```python
from build123d import *

# Parameters (mm, degrees)
F1_DEPTH = 18
F2_R     = 15
F4_D     = 8
F4_DEPTH = 15
F4_TIP   = 2.4034424761
F6_DEPTH = 18


# Not quite as in the source:
# - a feature names something its author has since deleted; it is built from what else it names


with BuildPart() as f1:
    # F0 (on Top) → F1 (new body)
    with BuildSketch(Plane.XY):
        Polygon((1700, 0), (0, 0), (0, -750), (1690, -750), (1700, -750), align=None)
    extrude(amount=F1_DEPTH)

    # F2
    f2_edges = [f1.edges().sort_by_distance(p)[0] for p in [
        (0, -750, 9),
        (0, 0, 9),
        (1700, 0, 9),
    ]]
    fillet(f2_edges, radius=F2_R)

    # F4
    with Locations(Plane(origin=(0, 0, 0), x_dir=(1, 0, 0), z_dir=(0, 0, -1))):
        with Locations((136.6116523517, 286.6116523517), (100, 250), (100, 375), (136.6116523517, 463.3883476483), (100, 500), (313.3883476483, 463.3883476483), (350, 375), (313.3883476483, 286.6116523517), (1200, 150), (1450, 150), (1589.5405845398, 110.4594154602), (1600, 250), (1450, 375), (1200, 375), (1417.1572875254, 467.1572875254), (1600, 500), (1593.933982822, 643.933982822), (1450, 650), (1200, 650), (1412.7638892432, 287.2361107568)):
            Hole(F4_D / 2, depth=F4_DEPTH)
            with Locations((0, 0, -(F4_DEPTH + F4_TIP / 2))):  # 118° drill point
                Cone(0, F4_D / 2, F4_TIP, mode=Mode.SUBTRACT)

    # F5 (on face) → F6 (cut)
    with BuildSketch(Plane(origin=(0, 0, 0), x_dir=(1, 0, 0), z_dir=(0, 0, -1))):
        with BuildLine():
            ThreePointArc((851.6666666667, 79.9826370047), (880.4880927062, 91.3965751745), (892.5, 119.973955507))
            ThreePointArc((892.5, 119.973955507), (824.5119072938, 148.5513358395), (851.6666666667, 79.9826370047))
        make_face()
    extrude(amount=-F6_DEPTH, mode=Mode.SUBTRACT)


solid = f1.part
```
Verification items for the finished model (mm, model axes). Coordinates: 2 decimals unless noted, no trailing zeros. Write each loop counter-clockwise with the first axis right and the second up, starting at its lowest first coordinate (ties: lowest second). Pieces come first, ordered by that corner, then holes. Notation, with made-up numbers: (45.25, 64) - (57.25, 64) arc R20 cw to (57.25, 90) - close; hole circle Ø1 at (56.5, -8). An arc over 180 degrees is marked (long way). One line per question, with ' | ' between items. Start each with the question number.
1. Draft check along X on faces 1 (the flat face through (838, -370, 0)), 2 (the cylindrical face through (823.02, -147.01, 8.87)). Enter one of: released by +X, released by -X, zero draft, split by the parting line, or undercut.
2. Material ranges on line 1 along X through (y, z) = (-650, 7); line 2 along Y through (x, z) = (1200, 6); line 3 along Y through (x, z) = (1603.5, 3.75), recorded low to high.
3. Section check A-A (x = 852.5). Enter the section's corners in (y, z).
4. Gauge pin test, flat end, axial feed: P1, Ø7, axis at x = 1417.16, y = -467.16, coming from the -Z side. Record the tip position at first contact, or that the pin passes through.
Computed values:
1) face 1: zero draft | face 2: undercut
2) line 1: 0 to 1196, 1204 to 1446, 1454 to 1700 | line 2: -750 to -654, -646 to -379, -371 to -154, -146 to 0 | line 3: -750 to -501.94, -498.06 to -251.94, -248.06 to 0
3) outline: (-750, 0) - (-159.97, 0) - (-159.97, 18) - (-750, 18) - close; (-79.97, 0) - (0, 0) - (0, 18) - (-79.97, 18) - close
4) P1: z = 15.3
